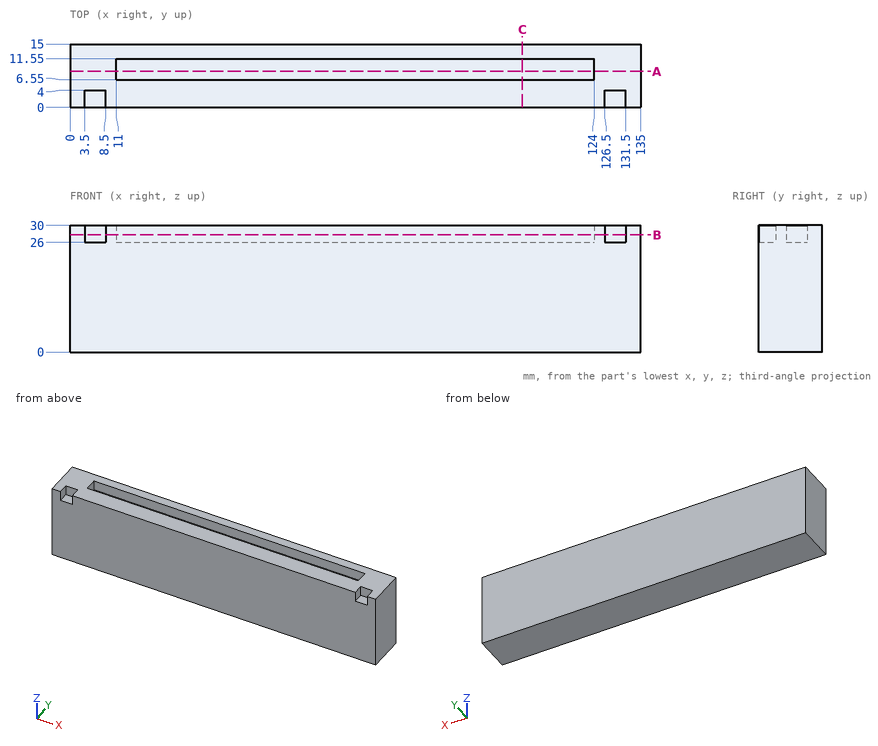
Geometry check sheet. Reference: drawing and pictorial views, mm from the part's lowest x, y, z. Round coordinates to 2 decimals unless told otherwise and drop trailing zeros. Loops run counter-clockwise (first coordinate to the right, second up) from the corner with the lowest first, then second, coordinate; pieces in that order, holes last. Notation, with made-up numbers: (67, 38.25) - (80, 38.25) arc R6 cw to (80, 48.25) - close; hole circle Ø3 at (-25.5, -12.5). An arc over 180 degrees is marked (long way). Write item = value, one per line. Start each with the question number.
Q1. Section check C-C (x = 107). Record the boundary of the cut face in (y, z), plus the area to 3 significant figures.
Q2. Section check A-A (y = 8.5). Record the boundary of the cut face in (x, z), plus the area to 3 significant figures.
Q3. Section check B-B (z = 27.75). Record the boundary of the cut face in (x, y).
Q4. Thickness scan on L1, parallel to Y at x = 123.5, z = 26.75; L2, parallel to Z at x = 57.5, y = 9. Record the ranges inside material, lowest first.
Q5. Depth check by flat-ended pin: P1, Ø1.2, axis at x = 128, z = 28, coming from the -Y side; P2, Ø2, axis at x = 130, y = 1, coming from the +Z side. Enter the tip coordinate at first touch or a pass-through.
Derived:
q1.outline = (0, 0) - (15, 0) - (15, 30) - (11.55, 30) - (11.55, 26) - (6.55, 26) - (6.55, 30) - (0, 30) - close
q1.area = 430 mm^2
q2.outline = (0, 0) - (135, 0) - (135, 30) - (124, 30) - (124, 26) - (11, 26) - (11, 30) - (0, 30) - close
q2.area = 3,600 mm^2
q3.outline = (0, 0) - (3.5, 0) - (3.5, 4) - (8.5, 4) - (8.5, 0) - (126.5, 0) - (126.5, 4) - (131.5, 4) - (131.5, 0) - (135, 0) - (135, 15) - (0, 15) - close; hole (11, 6.55) - (124, 6.55) - (124, 11.55) - (11, 11.55) - close
q4.L1 = 0 to 6.55, 11.55 to 15
q4.L2 = 0 to 26
q5.P1 = 4
q5.P2 = 26
